Read the model definition and answer for the solid it produces. Units are mm, in the model's axes. A direction names the side the tool comes from. Coordinates: 2 decimals unless noted, no trailing zeros. Loops run counter-clockwise (first coordinate to the right, second up) from the corner with the lowest first, then second, coordinate; pieces in that order, holes last. Notation, with made-up numbers: (-39.5, 47.25) -> (16.5, 47.25) arc R23 cw to (16.5, 81.25) -> close; hole circle Ø1 at (60, -9). An arc over 180 degrees is marked (long way). Answer as CSV lines item,"result".
Solid Edge part; units mm, degrees
sketch "Sketch1" plane through (0, 0, 58.9841) normal (0, 0, 1) x (1, 0, 0)
  arc A0 (-104.0747, 89.0237) -> (-104.0747, 98.9574) centre (-103.5, 93.9905) cw
  line L0 (-104.0747, 98.9574) -> (-82.6121, 101.4408)
  arc A1 (-82.6121, 101.4408) -> (-82.6121, 86.5402) centre (-81.75, 93.9905) cw
  line L1 (-82.6121, 86.5402) -> (-104.0747, 89.0237)
  circle A2 centre (-81.75, 93.9905) radius 3.6
  circle A3 centre (-103.5, 93.9905) radius 1.1
extrude "Protrusion1" add sketch "Sketch1" against normal blind 5
sketch "Sketch2" plane through (-91.375, 93.9905, 53.9841) normal (0, 0, -1) x (-0.9933721, 0.1149425, 0)
  circle A0 centre (2.856, -0.3304) radius 0.8
extrude "Cutout1" cut sketch "Sketch2" against normal through all
sketch "Sketch3" plane through (-91.375, 93.9905, 53.9841) normal (0, 0, -1) x (-0.9933721, 0.1149425, 0)
  line L0 (-8.7667, 4.6175) -> (4.8095, 1.5454)
  arc A0 (4.8095, 1.5454) -> (4.3293, -2.6027) centre (4.346, -0.5028) cw
  line L1 (4.3293, -2.6027) -> (-9.4884, -2.4929)
  arc A1 (-9.4884, -2.4929) -> (-8.7667, 4.6175) centre (-9.5612, 1.1063) cw
extrude "Cutout2" cut sketch "Sketch3" against normal blind 2
Q1. For faces 1 (the face through (-97.85, 93.95, 54.97)), 2 (the face through (-94.98, 94.32, 57.46)), determine the directions among +Z, -Z, +X, -X, +Y, -Y from which every point of the face is accessible in a straight line to the end or side of a thin tool.
Results:
face 1,"-Z"
face 2,"+Z, -Z"
Q2. For a pull along X with two mould halves and no side action, classify faces 3 (the face through (-91, 97, 53.984)), 4 (the face through (-108.5, 94.1, 56.5)), 5 (the face through (-90, 94, 55.984)), 6 (the face through (-88.958, 96.835, 54.97)) as pulls with the +X half, pulls with the -X half, needs draft (parallel to the pull), parting line crosses it, or undercut.
Results:
face 3,"needs draft"
face 4,"pulls with the -X half"
face 5,"undercut"
face 6,"undercut"
Q3. Find the intervals of material crossed by probe 1 along X at (y, z) = (93.5, 57.65); probe 2 along X at (y, z) = (93, 54.9); probe 3 along Z at (x, y) = (-87, 94.25), in increasing order. Write a range as [from, to].
Results:
probe 1,"x = [-108.48, -104.48], [-102.52, -94.88], [-93.62, -85.32], [-78.18, -74.27]"
probe 2,"x = [-108.4, -103.98], [-103.02, -97.6], [-78.29, -74.32]"
probe 3,"z = [55.98, 58.98]"
Q4. A cutting plane is placed at A-A, the plane x = -81.75. Write down the section's boundary in (y, z).
Results:
outline,"(86.49, 53.98) -> (90.39, 53.98) -> (90.39, 58.98) -> (86.49, 58.98) -> close; (97.59, 53.98) -> (101.49, 53.98) -> (101.49, 58.98) -> (97.59, 58.98) -> close"
Q5. A cutting plane is placed at D-D, the plane x = -86.5. Write down the section's boundary in (y, z), and give its area (3 significant figures).
Results:
outline,"(86.99, 53.98) -> (90.88, 53.98) -> (90.88, 55.98) -> (97.1, 55.98) -> (97.1, 53.98) -> (100.99, 53.98) -> (100.99, 58.98) -> (86.99, 58.98) -> close"
area,"57.6 mm²"
Q6. A cutting plane is placed at C-C, the plane z = 54.7. Give the number of separate pieces and of enclosed holes in the cut face, and give its area (3 significant figures).
Results:
separate pieces,"1"
enclosed holes,"2"
area,"290 mm²"
Q7. Given pin 1 Ø3.5 at (x, y) = (-87, 94.5) entering from -Z; pin 2 Ø2 at (x, y) = (-103.5, 93.99) entering from +Z; pin 3 Ø1.5 at (x, z) = (-83, 57.5) entering from -Y, each flat-ended and moving along its own axis, determine where each tip first touches the part or whether it passes through.
Results:
pin 1,"stops at z = 55.98"
pin 2,"passes through"
pin 3,"stops at y = 86.51"
Q8. A cutting plane is placed at B-B, the plane y = 95.75. Write down the section's boundary in (x, z), and give its area (3 significant figures).
Results:
outline,"(-108.18, 53.98) -> (-96.9, 53.98) -> (-96.9, 55.98) -> (-84.89, 55.98) -> (-84.89, 58.98) -> (-108.18, 58.98) -> close; (-78.61, 53.98) -> (-74.46, 53.98) -> (-74.46, 58.98) -> (-78.61, 58.98) -> close"
area,"113 mm²"
